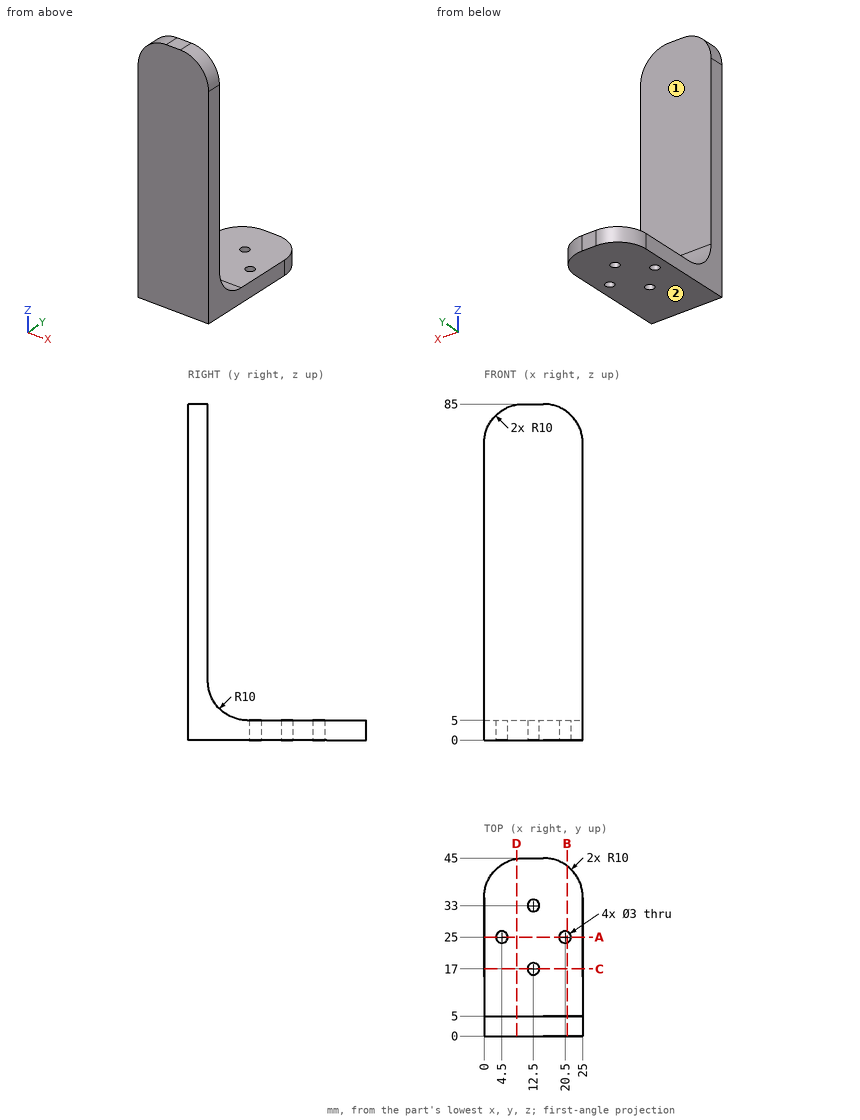
Input: dimensioned drawing with shaded views. Units: mm. Origin: part minimum x, y, z. A direction names the side the tool comes from. Round coordinates to 2 decimals unless told otherwise and drop trailing zeros. Loops run counter-clockwise (first coordinate to the right, second up) from the corner with the lowest first, then second, coordinate; pieces in that order, holes last. Notation, with made-up numbers: M -31,-22.75 L 11,-22.75 A21 cw 11,-5.75 Z; hole C 35,-3 d1. An arc over 180 degrees is marked long. Return JSON: item names as keys, results as strings. Group by question number.
1. Material intervals for line 1 along Y through (x, z) = (12.5, 2.3); line 2 along Y through (x, z) = (13, 80.5), sorted ascending. Write a range as from..to.
2. Pin query (flat end, axial travel): pin 1 (1.5 mm diameter, centred on x = 7.5, y = 8, fed in from +Z); pin 2 (1 mm diameter, centred on x = 19, z = 70, fed in from +Y); pin 3 (5 mm diameter, centred on x = 4.5, y = 25, fed in from +Z). Return the tip coordinate at first contact, or that it passes through.
3. Section query A-A on y = 25. Output: boundary loops of the cut face in (x, z), and give its area (3 significant figures).
4. Section query C-C on y = 17. Output: boundary loops of the cut face in (x, z), and give its area (3 significant figures).
5. Section query B-B on x = 21. Output: boundary loops of the cut face in (y, z), and give its area (3 significant figures).
6. Reachability of the marked faces 1 and 2 from +Z, -Z, +X, -X, +Y, -Y: full face, straight path, thin tool, end or side. Return the list, or none.
7. Section query D-D on x = 8.25. Output: boundary loops of the cut face in (y, z).
Checks:
{
 "1": {"line 1": "y = 0..15.5, 18.5..31.5, 34.5..45", "line 2": "y = 0..5"},
 "2": {"pin 1": "stops at z = 8.68", "pin 2": "stops at y = 5", "pin 3": "stops at z = 5"},
 "3": {"outline": "M 0,0 L 3,0 L 3,5 L 0,5 Z; M 6,0 L 19,0 L 19,5 L 6,5 Z; M 22,0 L 25,0 L 25,5 L 22,5 Z", "area": "95.0 mm²"},
 "4": {"outline": "M 0,0 L 11,0 L 11,5 L 0,5 Z; M 14,0 L 25,0 L 25,5 L 14,5 Z", "area": "110 mm²"},
 "5": {"outline": "M 0,0 L 23.59,0 L 23.59,5 L 15,5 A10 cw 5,15 L 5,83 L 0,83 Z; M 26.41,0 L 43,0 L 43,5 L 26.41,5 Z", "area": "612 mm²"},
 "6": {"face 1": "+Z, +X, -X, +Y", "face 2": "-Z, +X, -X, +Y, -Y"},
 "7": {"outline": "M 0,0 L 44.85,0 L 44.85,5 L 15,5 A10 cw 5,15 L 5,84.85 L 0,84.85 Z"}
}
